```python
from build123d import *

# Parameters (mm, degrees)
BOSS_EXTRUDE1_DEPTH      = 7.9
BOSS_EXTRUDE1_DEPTH_BACK = 7.9
FILLET1_RADIUS           = 7.9
FILLET1_LENGTH           = 1.2
CUT_EXTRUDE3_DEPTH       = 32.020477108
SKETCH5_R                = 3.2
CUT_EXTRUDE4_DEPTH       = 32.01273941
FILLET3_R                = 1


with BuildPart() as part:
    # Sketch3 → Boss-Extrude1 (new, two sides: drawn at the far end of the back side and taken through both)
    with BuildSketch(Plane(origin=(0, 0, 0), x_dir=(0, 0, -1), z_dir=(1, 0, 0)).offset(-BOSS_EXTRUDE1_DEPTH_BACK)):
        Polygon((0, 0), (-21.9, 0), (-21.9, 1.2), (-1.2, 1.2), (-1.2, 21.7), (0, 21.7), align=None)
    extrude(amount=BOSS_EXTRUDE1_DEPTH + BOSS_EXTRUDE1_DEPTH_BACK)

    # Fillet1: full round fillet: the end face becomes a half cylinder, R = half its width
    fillet1_face = Plane((0, 0.6, 21.9), x_dir=(0, -1, 0), z_dir=(0, 0, 1))  # on the end face: x along it, z out of the body
    fillet1_slab = fillet1_face.offset(-FILLET1_RADIUS / 2) * Box(FILLET1_LENGTH, 2 * FILLET1_RADIUS, FILLET1_RADIUS, mode=Mode.PRIVATE)  # the body's end, R deep
    fillet1_round = Plane((0, 0.6, 14), x_dir=(0, 0, 1), z_dir=(0, -1, 0)) * Cylinder(FILLET1_RADIUS, FILLET1_LENGTH, mode=Mode.PRIVATE)  # its axis R under the face
    add(fillet1_slab - fillet1_round, mode=Mode.SUBTRACT)

    # Sketch4 → Cut-Extrude3 (cut, through all)
    with BuildSketch(Plane(origin=(0, 1.2, 0), x_dir=(1, 0, 0), z_dir=(0, 1, 0))):
        with BuildLine():
            Line((-2.8, -8.490258859), (-2.8, -16.609741141))
            add(Edge.make_bspline(
                [(2.8, -16.629870216), (-0.006277243, -18.580174221), (-2.8, -16.609741141)],
                knots=[0, 0, 0, 1, 1, 1], degree=2))
            Line((2.8, -16.629870216), (2.8, -8.470129784))
            add(Edge.make_bspline(
                [(2.8, -8.470129784), (-0.006277243, -6.519825779), (-2.8, -8.490258859)],
                knots=[0, 0, 0, 1, 1, 1], degree=2))
        make_face()
    extrude(amount=-CUT_EXTRUDE3_DEPTH, mode=Mode.SUBTRACT)

    # Sketch5 → Cut-Extrude4 (cut, through all)
    with BuildSketch(Plane.XY.offset(1.2)):
        with Locations((0, 9.7)):
            Circle(SKETCH5_R)
    extrude(amount=-CUT_EXTRUDE4_DEPTH, mode=Mode.SUBTRACT)

    # Fillet3
    fillet3_edges = [part.edges().sort_by_distance(p)[0] for p in [
        (0, 0, 0),
    ]]
    fillet(fillet3_edges, radius=FILLET3_R)


solid = part.part
```
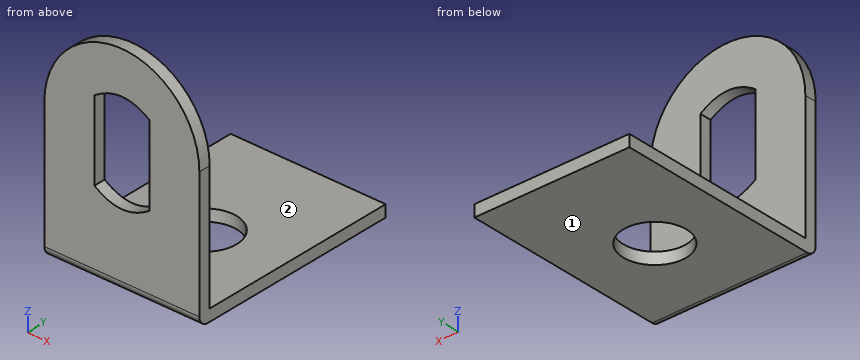
Read the model definition and answer for the solid it produces. Units are mm, in the model's axes. Face numbers are marked on the shaded views. A direction names the side the tool comes from. Coordinates: 2 decimals unless noted, no trailing zeros. Write each loop counter-clockwise with the first axis right and the second up, starting at its lowest first coordinate (ties: lowest second). Pieces come first, ordered by that corner, then holes. Notation, with made-up numbers: (-34.5, 46) - (2.5, 46) arc R6 ccw to (2.5, 52) - close; hole circle Ø5 at (5.5, -20.75). An arc over 180 degrees is marked (long way). Answer as a JSON object with one key per item and string values. Group by question number.
1. A cutting plane is placed at D-D (x = -4.5). Determine the outline of the cut face in (y, z), plus the area to 3 significant figures.
2. Consider L1, parallel to Y at x = 0, z = 0.9; L2, parallel to Y at x = -2.75, z = 7. Determine where each line is inside the solid, lowest interval first. Write a range as [from, to].
3. A cutting plane is placed at B-B (z = 9.75). Determine the outline of the cut face in (x, y).
4. Which of the six approach directions +Z, -Z, +X, -X, +Y, -Y give full straight-line access (tool end or side, diameter ignored) to the marked faces 1 and 2?
5. A cutting plane is placed at C-C (x = 0). Give the number of separate pieces and of enclosed holes in the cut face, plus the area to 3 significant figures.
6. Each of these flat-tipped pins is pushed along its axis until it touches: P1, Ø1, axis at x = -0.5, z = 8, coming from the +Y side; P2, Ø5, axis at x = 0, y = 9.7, coming from the +Z side; P3, Ø4, axis at x = 3, y = 3.5, coming from the +Z side. Where does it stop, or does it pass through?
7. A cutting plane is placed at A-A (y = 9.7). Determine the outline of the cut face in (x, z).
Worked out:
{
 "1": {"outline": "(0, 1) arc R1 ccw to (1, 0) - (21.7, 0) - (21.7, 1.2) - (1.2, 1.2) - (1.2, 20.49) - (0, 20.49) - close", "area": "49.0 mm²"},
 "2": {"L1": "y = [0.01, 6.5], [12.9, 21.7]", "L2": "y = [0, 1.2]"},
 "3": {"outline": "(-7.9, 0) - (-2.8, 0) - (-2.8, 1.2) - (-7.9, 1.2) - close; (2.8, 0) - (7.9, 0) - (7.9, 1.2) - (2.8, 1.2) - close"},
 "4": {"face 1": "-Z, +X, -X, +Y, -Y", "face 2": "+Z, +X, -X, +Y"},
 "5": {"separate pieces": "3", "enclosed holes": "0", "area": "30.9 mm²"},
 "6": {"P1": "stops at y = 1.2", "P2": "passes through", "P3": "stops at z = 1.2"},
 "7": {"outline": "(-7.9, 0) - (-3.2, 0) - (-3.2, 1.2) - (-7.9, 1.2) - close; (3.2, 0) - (7.9, 0) - (7.9, 1.2) - (3.2, 1.2) - close"}
}
